Input: part model. Units: mm. Frame: model coordinates. A direction names the side the tool comes from. Round coordinates to 2 decimals unless told otherwise and drop trailing zeros. Order: outer loops, then holes, each group sorted by start corner. A loop starts at its lowest first (then second) coordinate and runs counter-clockwise, first axis right, second up.
Item 1: Cut plane B-B on z = 1.6. Give the number of separate pieces and of enclosed holes in the cut face, then the cut area to 3 significant figures.
Item 2: First-contact query: pin 1 (0.8 mm diameter, centred on y = -5.5, z = 1.5, fed in from -X); pin 2 (0.9 mm diameter, centred on x = -26.5, z = 2, fed in from +Y); pin 3 (1.5 mm diameter, centred on x = -25, z = 1, fed in from -Y). Flat tips, straight axial feed; report the tip coordinate or a pass-through.
Item 3: Cut plane C-C on x = 11. Output: boundary loops of the cut face in (y, z).
Item 4: Reachability of faces 5 (the flat face through (63, -10, 1)), 6 (the cylindrical face through (-41.73, -10.76, 1.48)), 7 (the flat face through (24, -5.5, 1)), 8 (the flat face through (-65, -8.5, 1)), 9 (the cylindrical face through (-41.63, 10.72, 1.48)) from +Z, -Z, +X, -X, +Y, -Y: full face, straight path, thin tool, end or side. Return the list, or none.
Item 5: Mould query, pull axis X, two halves, no side actions, for faces 1 (the flat face through (-2, 0, 3)), 2 (the flat face through (19.565, 2.712, 1.479)), 3 (the flat face through (-19.903, 3.296, 1.479)), 4 (the flat face through (-48.43, -2.46, 1.48)). Classes: released by +X, released by -X, zero draft, split by the parting line, or undercut.
Item 6: Line query: L1, parallel to X at y = 0, z = 2.25; L2, parallel to Y at x = -22, z = 0.95; L3, parallel to X at y = 0.5, z = 1.8. Output: solid intervals per line, ascending.
Item 7: Cut plane A-A on x = -54. Output: boundary loops of the cut face in (y, z).
```python
from build123d import *

# Parameters (mm, degrees)
F1_DEPTH = 3


with BuildPart() as f1:
    # F0 (on Top) → F1 (new body)
    with BuildSketch(Plane.XY):
        with BuildLine():
            ThreePointArc((-37.904082, 10), (-41.683727, 10.741799), (-44.902624, 12.857143))
            ThreePointArc((-44.902624, 12.857143), (-60.223634, 17.792746), (-73.366632, 8.5))
            Line((-73.366632, 8.5), (-57.671361, 8.5))
            ThreePointArc((-57.671361, 8.5), (-56.257147, 7.914214), (-55.671361, 6.5))
            Line((-55.671361, 6.5), (-55.671361, 5))
            Line((-55.671361, 5), (-52.78461, 5))
            Line((-52.78461, 5), (-49.897858, 5))
            Line((-49.897858, 5), (-47.011107, 0))
            Line((-47.011107, 0), (-49.897858, -5))
            Line((-49.897858, -5), (-52.78461, -5))
            Line((-52.78461, -5), (-55.671361, -5))
            Line((-55.671361, -5), (-55.671361, -6.5))
            ThreePointArc((-55.671361, -6.5), (-56.257147, -7.914214), (-57.671361, -8.5))
            Line((-57.671361, -8.5), (-73.366632, -8.5))
            ThreePointArc((-73.366632, -8.5), (-60.223634, -17.792746), (-44.902624, -12.857143))
            ThreePointArc((-44.902624, -12.857143), (-41.683727, -10.741799), (-37.904082, -10))
            Line((-37.904082, -10), (39.611456, -10))
            ThreePointArc((39.611456, -10), (43.179677, -10.658276), (46.278123, -12.54644))
            ThreePointArc((46.278123, -12.54644), (59.221926, -16.744511), (71.040446, -10))
            Line((71.040446, -10), (54.285218, -10))
            ThreePointArc((54.285218, -10), (53.172521, -9.661898), (52.436029, -8.761905))
            ThreePointArc((52.436029, -8.761905), (50.701706, 0), (52.436029, 8.761905))
            ThreePointArc((52.436029, 8.761905), (53.172521, 9.661898), (54.285218, 10))
            Line((54.285218, 10), (71.040446, 10))
            ThreePointArc((71.040446, 10), (59.221926, 16.744511), (46.278123, 12.54644))
            ThreePointArc((46.278123, 12.54644), (43.179677, 10.658276), (39.611456, 10))
            Line((39.611456, 10), (-37.904082, 10))
        make_face()
        Polygon((-33.011107, 0), (-29.25833, 6.5), (-21.752777, 6.5), (-18, 0), (-21.752777, -6.5), (-29.25833, -6.5), align=None, mode=Mode.SUBTRACT)
        Polygon((18, 0), (21.175426, 5.5), (27.526279, 5.5), (30.701706, 0), (27.526279, -5.5), (21.175426, -5.5), align=None, mode=Mode.SUBTRACT)
    extrude(amount=F1_DEPTH)


solid = f1.part
```
From the geometry:
1. separate pieces: 1
1. enclosed holes: 2
1. area: 2,480 mm2
2. pin 1: stops at x = -55.67
2. pin 2: stops at y = 10
2. pin 3: stops at y = -10
3. outline: (-10, 0) - (10, 0) - (10, 3) - (-10, 3) - close
4. face 5: +Z, -Z, +X
4. face 6: +Z, -Z, -Y
4. face 7: +Z, -Z
4. face 8: +Z, -Z, -X
4. face 9: +Z, -Z, +Y
5. face 1: zero draft
5. face 2: undercut
5. face 3: undercut
5. face 4: released by -X
6. L1: x = -47.01 to -33.01, -18 to 18, 30.7 to 50.7
6. L2: y = -10 to -6.5, 6.5 to 10
6. L3: x = -47.3 to -32.72, -18.29 to 18.29, 30.41 to 50.71
7. outline: (-17.66, 0) - (-5, 0) - (-5, 3) - (-17.66, 3) - close; (5, 0) - (17.66, 0) - (17.66, 3) - (5, 3) - close
